```python
from build123d import *

# Parameters (mm, degrees)
USB_LIP_DEPTH                       = 1.55
BASE_START                          = -1.1
SKETCH1_3_W                         = 18.28
SKETCH1_3_H                         = 20.828
BASE_W_1_1MM_COMPONENT_OFFSET_DEPTH = 1
SKETCH1_4_W                         = 3
SKETCH1_4_H                         = 20.828
SIDES_DEPTH                         = 2.1
SKETCH2_W                           = 7.54
SKETCH2_H                           = 0.9
USB_SIDES_DEPTH                     = 3.4
SKETCH3_W                           = 24.28
SKETCH3_H                           = 0.9
USB_TOP_DEPTH                       = 0.95
SKETCH4_W                           = 3
SKETCH4_H                           = 11.414
SIDE_GUARDS_DEPTH                   = 5.9
SKETCH5_R                           = 0.9
MOUNT_HOLES_DEPTH                   = 32.447486132


with BuildPart() as part:
    # Sketch1 → USB Lip (new body)
    with BuildSketch(Plane(origin=(0, 0, 0), x_dir=(1, 0, 0), z_dir=(0, 1, 0))):
        Polygon((18.28, 20.828), (21.28, 20.828), (21.28, 21.728), (-3, 21.728), (-3, 20.828), (0, 20.828), align=None)
    extrude(amount=USB_LIP_DEPTH)



with BuildPart() as body_2:
    # Sketch1<3> → Base w/ 1.1mm component offset (new body)
    with BuildSketch(Plane(origin=(0, 0, 0), x_dir=(1, 0, 0), z_dir=(0, 1, 0)).offset(BASE_START)):
        with Locations((9.14, 10.414)):
            Rectangle(SKETCH1_3_W, SKETCH1_3_H)
    extrude(amount=-BASE_W_1_1MM_COMPONENT_OFFSET_DEPTH)


with BuildPart() as part_1:
    add(part.part)

    add(body_2.part)  # Sides merges body 2
    # Sketch1<4> → Sides (add)
    with BuildSketch(Plane(origin=(0, 0, 0), x_dir=(1, 0, 0), z_dir=(0, 1, 0))):
        with Locations((-1.5, 10.414)):
            Rectangle(SKETCH1_4_W, SKETCH1_4_H)
        Polygon((21.28, 0), (21.28, -1), (-3, -1), (-3, 0), (0, 0), (18.28, 0), align=None)
        with Locations((19.78, 10.414)):
            Rectangle(SKETCH1_4_W, SKETCH1_4_H)
        Polygon((18.28, 20.828), (21.28, 20.828), (21.28, 21.728), (-3, 21.728), (-3, 20.828), (0, 20.828), align=None)
    extrude(amount=-SIDES_DEPTH)

    # Sketch2 → USB Sides (add)
    with BuildSketch(Plane(origin=(0, 1.55, 0), x_dir=(1, 0, 0), z_dir=(0, 1, 0))):
        with Locations((0.77, 21.278)):
            Rectangle(SKETCH2_W, SKETCH2_H)
        with Locations((17.51, 21.278)):
            Rectangle(SKETCH2_W, SKETCH2_H)
    extrude(amount=USB_SIDES_DEPTH)

    # Sketch3 → USB Top (add)
    with BuildSketch(Plane(origin=(0, 4.95, 0), x_dir=(1, 0, 0), z_dir=(0, 1, 0))):
        with Locations((9.14, 21.278)):
            Rectangle(SKETCH3_W, SKETCH3_H)
    extrude(amount=USB_TOP_DEPTH)

    # Sketch4 → Side Guards (add)
    with BuildSketch(Plane(origin=(0, 0, 0), x_dir=(1, 0, 0), z_dir=(0, 1, 0))):
        with Locations((-1.5, 4.707)):
            Rectangle(SKETCH4_W, SKETCH4_H)
        with Locations((19.78, 4.707)):
            Rectangle(SKETCH4_W, SKETCH4_H)
    extrude(amount=SIDE_GUARDS_DEPTH)

    # Sketch5 → Mount Holes (cut, through all)
    with BuildSketch(Plane(origin=(0, 5.9, 0), x_dir=(1, 0, 0), z_dir=(0, 1, 0))):
        with Locations(Location((-1.5, 2, 0), (0, 0, 270))):
            Circle(SKETCH5_R)
        with Locations(Location((19.78, 2, 0), (0, 0, 270))):
            Circle(SKETCH5_R)
        with Locations(Location((-1.5, 7, 0), (0, 0, 270))):
            Circle(SKETCH5_R)
        with Locations(Location((19.78, 7, 0), (0, 0, 270))):
            Circle(SKETCH5_R)
    extrude(amount=-MOUNT_HOLES_DEPTH, mode=Mode.SUBTRACT)


solid = part_1.part
```
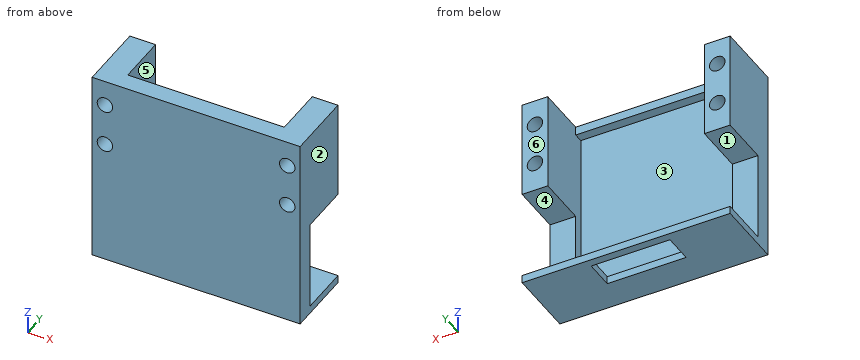
Part model, mm, in its own coordinate system. Face numbers are marked on the shaded views. A direction names the side the tool comes from. Round coordinates to 2 decimals unless told otherwise and drop trailing zeros. Order: outer loops, then holes, each group sorted by start corner. A loop starts at its lowest first (then second) coordinate and runs counter-clockwise, first axis right, second up. Notation, with made-up numbers: M 6,70.5 L 58,70.5 A16 ccw 58,90.5 Z; hole C 38.5,28 d4. An arc over 180 degrees is marked long. Answer in a Markdown table with one row per item. Add a question column.
Q1. Cut at C-C on x = 13. Give the cut face in (y, z), and give its area (3 significant figures).
Q2. Mould opens along X. For the marked faces 1, 2 and 3 say: +X half, -X half, draft (parallel to the pull), parting line (faces both ways), or undercut.
Q3. 3-axis set-ups, long thin cutter, end or side, ignore diameter. For the marked faces 4, 5 and 6: which of +Z, -Z, +X, -X, +Y, -Y reach the whole face in a straight line?
Q4. Pin check, flat tips, straight feed: pin 1 (2.5 mm diameter, centred on x = -1.5, z = -7, fed in from +Y); pin 2 (3.5 mm diameter, centred on x = 13, y = 3.5, fed in from +Z); pin 3 (1.5 mm diameter, centred on x = -1.5, z = -14.5, fed in from +Y); pin 4 (1 mm diameter, centred on x = 13.5, z = -17, fed in from +Y). Stop position of each tip, or through.
Q5. Cut at D-D on y = 3. Give the cut face in (x, z).
Q6. Cut at B-B on z = -7. Give the cut face in (x, y), and give its area (3 significant figures).
Q7. Wall check: L1, parallel to X at y = 4, z = -7; L2, parallel to X at y = 1.5, z = -1; L3, parallel to Y at x = 12, z = -13.5. Give the ranges that are in metal, low to high. Write a range as from..to.
Q8. Cut at A-A on y = 0.75. Give the cut face in (x, z), and give its area (3 significant figures).
Established:
| question | item | result |
|---|---|---|
| 1 | outline | M -2.1,-21.73 L 1.55,-21.73 L 1.55,-20.83 L -1.1,-20.83 L -1.1,0 L 0,0 L 0,1 L -2.1,1 Z; M 4.95,-21.73 L 5.9,-21.73 L 5.9,-20.83 L 4.95,-20.83 Z |
| 1 | area | 27.1 mm2 |
| 2 | face 1 | draft |
| 2 | face 2 | +X half |
| 2 | face 3 | undercut |
| 3 | face 4 | +X, -X, +Y |
| 3 | face 5 | +Y |
| 3 | face 6 | +Z, -Z, +X, -X, +Y |
| 4 | pin 1 | stops at y = 5.9 |
| 4 | pin 2 | stops at z = -20.83 |
| 4 | pin 3 | stops at y = 0 |
| 4 | pin 4 | stops at y = -1.1 |
| 5 | outline | M -3,-21.73 L 4.54,-21.73 L 4.54,-20.83 L -3,-20.83 Z; M -3,-10.41 L 0,-10.41 L 0,1 L -3,1 Z; M 13.74,-21.73 L 21.28,-21.73 L 21.28,-20.83 L 13.74,-20.83 Z; M 18.28,-10.41 L 21.28,-10.41 L 21.28,1 L 18.28,1 Z; hole C -1.5,-7 d1.8; hole C -1.5,-2 d1.8; hole C 19.78,-7 d1.8; hole C 19.78,-2 d1.8 |
| 6 | outline | M -3,-2.1 L -2.4,-2.1 L -2.4,5.9 L -3,5.9 Z; M -0.6,-2.1 L 18.88,-2.1 L 18.88,5.9 L 18.28,5.9 L 18.28,-1.1 L 0,-1.1 L 0,5.9 L -0.6,5.9 Z; M 20.68,-2.1 L 21.28,-2.1 L 21.28,5.9 L 20.68,5.9 Z |
| 6 | area | 37.5 mm2 |
| 7 | L1 | x = -3..-2.4, -0.6..0, 18.28..18.88, 20.68..21.28 |
| 7 | L2 | x = -3..0, 18.28..21.28 |
| 7 | L3 | y = -2.1..-1.1 |
| 8 | outline | M -3,-21.73 L 21.28,-21.73 L 21.28,-20.83 L -3,-20.83 Z; M -3,-10.41 L 0,-10.41 L 0,1 L -3,1 Z; M 18.28,-10.41 L 21.28,-10.41 L 21.28,1 L 18.28,1 Z; hole C -1.5,-7 d1.8; hole C -1.5,-2 d1.8; hole C 19.78,-7 d1.8; hole C 19.78,-2 d1.8 |
| 8 | area | 80.2 mm2 |
